For this review, take the finished solid that the model builds, in its own axes (mm). A direction names the side the tool comes from. Coordinates: 2 decimals unless noted, no trailing zeros. Write each loop counter-clockwise with the first axis right and the second up, starting at its lowest first coordinate (ties: lowest second). Pieces come first, ordered by that corner, then holes. Notation, with made-up numbers: M 5.25,34 L 13.25,34 A18 ccw 13.25,48 Z; hole C -13,57.25 d1. An arc over 180 degrees is marked long. Return JSON: item names as keys, results as strings.
```python
from build123d import *

# Parameters (mm, degrees)
F2_SIZE = 0.254
F4_D    = 5.1054


with BuildPart() as f1:
    # F0 (on Front) → F1 (revolve)
    with BuildSketch(Plane.XZ):
        Polygon((11.303, 6.3881), (3.175, 6.3881), (3.175, 7.47395), (0, 7.47395), (0, 0), (22.86, 0), (25.4, 0), (25.4, 6.3881), (13.68425, 6.3881), (13.68425, 4.00685), (11.303, 4.00685), align=None)
    revolve(axis=Axis((11.43, 0, 0), (1, 0, 0)))

    # F2
    f2_edges = [f1.edges().sort_by_distance(p)[0] for p in [
        (0, 0, -7.47395),
        (25.4, 0, -6.3881),
        (13.68425, 0, -6.3881),
    ]]
    chamfer(f2_edges, length=F2_SIZE)

    # F4 (through all)
    with Locations(Plane.YZ.offset(25.4)):
        with Locations((0, 0)):
            Hole(F4_D / 2)


solid = f1.part
```
1. We need section A-A (y = 0). State the section outline as (x, z) points (3 decimals).
Checks:
{"outline": "M 0,-7.22 L 0.254,-7.474 L 3.175,-7.474 L 3.175,-6.388 L 11.303,-6.388 L 11.303,-4.007 L 13.684,-4.007 L 13.684,-6.134 L 13.938,-6.388 L 25.146,-6.388 L 25.4,-6.134 L 25.4,-2.553 L 0,-2.553 Z; M 0,2.553 L 25.4,2.553 L 25.4,6.134 L 25.146,6.388 L 13.938,6.388 L 13.684,6.134 L 13.684,4.007 L 11.303,4.007 L 11.303,6.388 L 3.175,6.388 L 3.175,7.474 L 0.254,7.474 L 0,7.22 Z"}
2. Clearance check with flat-ended pins moving along their axes: pin 1 Ø1.5 at (x, y) = (18.5, 1.5) entering from -Z; pin 2 Ø3 at (y, z) = (0, 0) entering from -X; pin 3 Ø8 at (x, z) = (18, 2.5) entering from -Y; pin 4 Ø6 at (x, y) = (15, -1) entering from +Z. State where each tip first meets the part, or that it passes through.
Checks:
{"pin 1": "z = -6.34", "pin 2": "through", "pin 3": "y = -6.39", "pin 4": "z = 6.39"}
3. For faces 4 (the face through (19.5, -1.9, 6.1)), 5 (the face through (12.477, 1.535, 3.701)), 6 (the face through (1.7, 7.3, -1.6)), list the 3-axis set-ups (+Z, -Z, +X, -X, +Y, -Y) from which the entire face can be reached by the end or side of a thin tool; tool diameter is ignored.
Checks:
{"face 4": "+X", "face 5": "none", "face 6": "+X, -X"}
4. Draft analysis for pull direction X (two halves, no side actions). For faces 1 (the face through (0, 0, 3)), 2 (the face through (25.4, 3, 0)), 3 (the face through (11.303, -3, -3)), state which applies: +X half, -X half, draft (parallel to the pull), parting line (faces both ways), or undercut.
Checks:
{"face 1": "-X half", "face 2": "+X half", "face 3": "undercut"}
5. We need section C-C (x = 22.5). State the section outline as (y, z) points.
Checks:
{"outline": "C 0,0 d12.78; hole C 0,0 d5.11"}
6. Wall thickness on L1, parallel to Z at x = 19.5, y = 0; L2, parallel to X at y = 3.75, z = -3.5; L3, parallel to Y at x = 22.75, z = 0.75: over which ranges is each line inside the solid? List them lowest first. Write a range as from..to.
Checks:
{"L1": "-6.39..-2.55, 2.55..6.39", "L2": "0..11.3, 13.68..25.4", "L3": "-6.34..-2.44, 2.44..6.34"}
